The listing builds one solid part. Answer for the finished solid, in the listing's coordinates (mm). Round coordinates to 2 decimals unless told otherwise and drop trailing zeros. Write each loop counter-clockwise with the first axis right and the second up, starting at its lowest first coordinate (ties: lowest second). Pieces come first, ordered by that corner, then holes. Notation, with made-up numbers: M 72,51 L 119,51 A18 ccw 119,64 Z; hole C 16,-38.75 d1. An arc over 180 degrees is marked long. Answer as CSV lines item,"result". Start each with the question number.
from build123d import *

# Parameters (mm, degrees)
F0_R     = 1.778
F0_R_2   = 6.35
F1_DEPTH = 6.35


with BuildPart() as f1:
    # F0 (on Front) → F1 (new body)
    with BuildSketch(Plane.XZ):
        with BuildLine():
            ThreePointArc((127.545797, 53.804597), (103.389041, -92.052002), (-38.696128, -132.911529))
            Line((-38.696128, -132.911529), (-46.095596, -151.796758))
            Line((-46.095596, -151.796758), (-38.616359, -151.796758))
            Line((-38.616359, -151.796758), (200.989076, -151.796758))
            Line((200.989076, -151.796758), (200.989076, -145.446758))
            Line((200.989076, -145.446758), (200.989076, 53.804597))
            Line((200.989076, 53.804597), (127.545797, 53.804597))
        make_face()
        with Locations((51.796343, -140.985444)):
            Circle(F0_R, mode=Mode.SUBTRACT)
        with Locations((87.590314, -141.603768)):
            Circle(F0_R, mode=Mode.SUBTRACT)
        with Locations((162.381076, -142.525758)):
            Circle(F0_R, mode=Mode.SUBTRACT)
        with Locations((152.602076, -132.746758)):
            Circle(F0_R, mode=Mode.SUBTRACT)
        with Locations((162.381076, -132.746758)):
            Circle(F0_R_2, mode=Mode.SUBTRACT)
        with Locations((181.939076, -142.525758)):
            Circle(F0_R, mode=Mode.SUBTRACT)
        with Locations((172.160076, -132.746758)):
            Circle(F0_R, mode=Mode.SUBTRACT)
        with Locations((181.939076, -132.746758)):
            Circle(F0_R_2, mode=Mode.SUBTRACT)
        with Locations((191.718076, -132.746758)):
            Circle(F0_R, mode=Mode.SUBTRACT)
        with Locations((162.381076, -122.967758)):
            Circle(F0_R, mode=Mode.SUBTRACT)
        with Locations((161.235617, -113.188758)):
            Circle(F0_R, mode=Mode.SUBTRACT)
        with Locations((181.939076, -122.967758)):
            Circle(F0_R, mode=Mode.SUBTRACT)
        with Locations((171.014617, -113.188758)):
            Circle(F0_R_2, mode=Mode.SUBTRACT)
        with Locations((180.793617, -113.188758)):
            Circle(F0_R, mode=Mode.SUBTRACT)
        with Locations((171.014617, -103.409758)):
            Circle(F0_R, mode=Mode.SUBTRACT)
        with Locations((178.707197, 44.601519)):
            Circle(F0_R, mode=Mode.SUBTRACT)
    extrude(amount=F1_DEPTH)


solid = f1.part
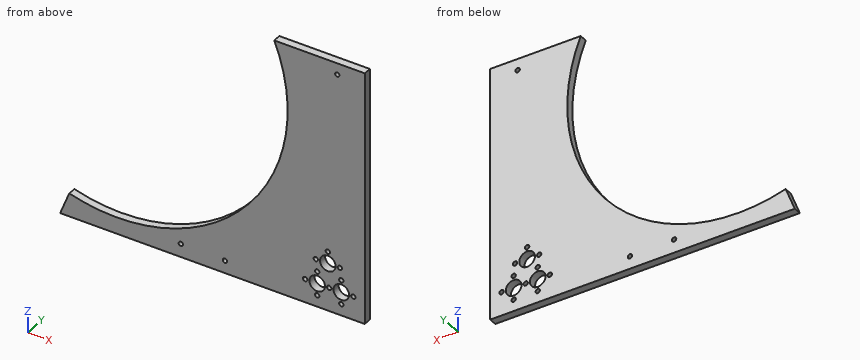
Q1. Straight lines are drawn through the part: L1, parallel to X at y = -2.75, z = -143; L2, parallel to X at y = -6, z = -109.5; L3, parallel to Z at x = 159, y = -5.25. For each, find the intervals that lie inside material, in ascending order.
Q2. Find section A-A (y = -1). Count the separate pieces of the cut face and the enclosed holes in it, plus the area to 3 significant figures.
Q3. Find section C-C (x = 75). Determine the outline of the cut face in (y, z).
Q4. Find section B-B (z = 19). Determine the outline of the cut face in (x, y).
Reported:
1,L1,"x = -42.65 to 86.49, 88.69 to 160.67, 164.09 to 180.23, 183.65 to 200.99"
1,L2,"x = 84.69 to 165.85, 176.18 to 200.99"
1,L3,"z = -151.8 to -138.12, -127.37 to 53.8"
2,separate pieces,"1"
2,enclosed holes,"16"
2,area,"19,200 mm2"
3,outline,"M -6.35,-151.8 L 0,-151.8 L 0,-116.35 L -6.35,-116.35 Z"
4,outline,"M 137.12,-6.35 L 200.99,-6.35 L 200.99,0 L 137.12,0 Z"
